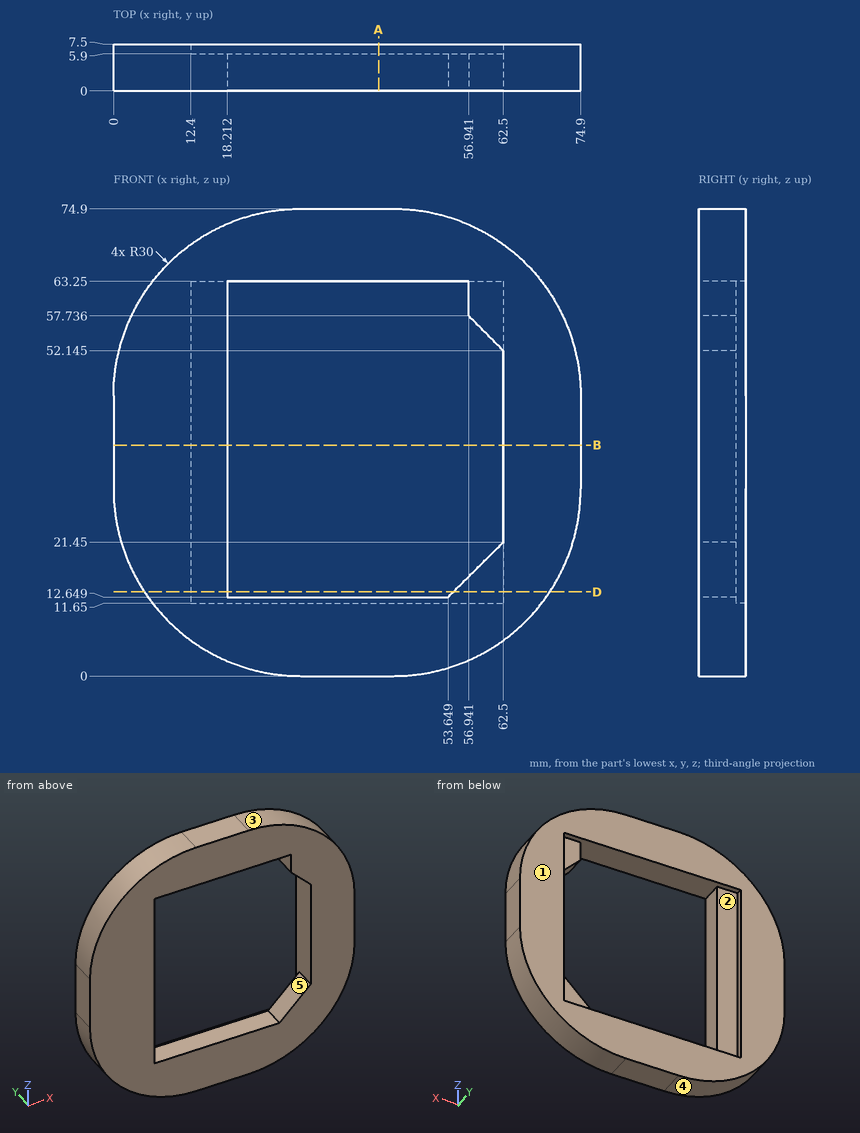
Drawing for the job (mm, zero at the part's lowest x, y, z). A direction names the side the tool comes from. Round coordinates to 2 decimals unless told otherwise and drop trailing zeros. Loops run counter-clockwise (first coordinate to the right, second up) from the corner with the lowest first, then second, coordinate; pieces in that order, holes last. Notation, with made-up numbers: M 68,10 L 125,10 A17 cw 125,20 Z; hole C 15,38.5 d7. An arc over 180 degrees is marked long. Use a Markdown table: item, result. Add a question column.
(1) Drill centre lines: line 1 (Z direction, x = 35, y = 4); line 2 (X direction, y = 1.25, z = 32); line 3 (X direction, y = 4.5, z = 50). Where is each one in solid material? Low to high.
(2) Cut at A-A (x = 42.5). Give the cut face in (y, z), and give its area (3 significant figures).
(3) Which spindle directions (+Z, -Z, +X, -X, +Y, -Y) get a long thin tool onto all of the face, cutting with end or side? Do the marked faces 1 and 2. Say none if no direction does.
(4) Cut at B-B (z = 37). Give the cut face in (x, y), and give its area (3 significant figures).
(5) Flat gauge pins, fed straight in: pin 1 (4 mm diameter, centred on x = 27, y = 4.5, fed in from -Z); pin 2 (2 mm diameter, centred on x = 13.5, z = 51, fed in from +Y); pin 3 (4.5 mm diameter, centred on y = 2, z = 59.5, fed in from -X). Where does each tip first touch, or does it go through?
(6) Cut at D-D (z = 13.5). Give the cut face in (x, y) (1 decimal), and give its area (3 significant figures).
(7) Pull direction X, two halves, no side cores. Call the marked faces 3, 4 and 5: +X half, -X half, draft (parallel to the pull), parting line (faces both ways), or undercut.
Geometry says:
| question | item | result |
|---|---|---|
| 1 | line 1 | z = 0 to 12.65, 63.25 to 74.9 |
| 1 | line 2 | x = 0 to 18.21, 62.5 to 74.9 |
| 1 | line 3 | x = 0.44 to 18.21, 62.5 to 74.46 |
| 2 | outline | M 0,0 L 7.5,0 L 7.5,11.65 L 5.9,11.65 L 5.9,12.65 L 0,12.65 Z; M 0,63.25 L 7.5,63.25 L 7.5,74.9 L 0,74.9 Z |
| 2 | area | 181 mm² |
| 3 | face 1 | +Z, -Z, +X, -X, +Y |
| 3 | face 2 | +Y |
| 4 | outline | M 0,0 L 18.21,0 L 18.21,5.9 L 12.4,5.9 L 12.4,7.5 L 0,7.5 Z; M 62.5,0 L 74.9,0 L 74.9,7.5 L 62.5,7.5 Z |
| 4 | area | 220 mm² |
| 5 | pin 1 | stops at z = 0.02 |
| 5 | pin 2 | stops at y = 5.9 |
| 5 | pin 3 | stops at x = 2.66 |
| 6 | outline | M 4.9,0 L 18.2,0 L 18.2,5.9 L 12.4,5.9 L 12.4,7.5 L 4.9,7.5 Z; M 54.5,0 L 70,0 L 70,7.5 L 62.5,7.5 L 62.5,5.9 L 54.5,5.9 Z |
| 6 | area | 193 mm² |
| 7 | face 3 | +X half |
| 7 | face 4 | -X half |
| 7 | face 5 | undercut |
